Source: CAD feature listing. Evaluate the final solid. Frame: model axes, mm. Coordinates: 2 decimals unless noted, no trailing zeros. Order: outer loops, then holes, each group sorted by start corner. A loop starts at its lowest first (then second) coordinate and runs counter-clockwise, first axis right, second up.
```python
from build123d import *

# Parameters (mm, degrees)
SKETCH_R  = 1.8288
PAD_DEPTH = 3


with BuildPart() as part:
    # Sketch → Pad (new body)
    with BuildSketch(Plane.XY):
        with BuildLine():
            Line((0, 126), (0, 1))
            ThreePointArc((0, 1), (0.292893, 0.292893), (1, 0))
            Line((1, 0), (14.748, 0))
            ThreePointArc((14.748, 0), (15.455107, 0.292893), (15.748, 1))
            Line((15.748, 12.7), (15.748, 1))
            ThreePointArc((22.352, 12.7), (19.05, 16.002), (15.748, 12.7))
            Line((22.352, 12.7), (22.352, 1))
            ThreePointArc((22.352, 1), (22.644893, 0.292893), (23.352, 0))
            Line((23.352, 0), (150.6479, 0))
            ThreePointArc((150.6479, 0), (151.355007, 0.292893), (151.6479, 1))
            Line((151.6479, 12.7), (151.6479, 1))
            ThreePointArc((158.2519, 12.7), (154.9499, 16.002), (151.6479, 12.7))
            Line((158.2519, 12.7), (158.2519, 1))
            ThreePointArc((158.2519, 1), (158.544793, 0.292893), (159.2519, 0))
            Line((159.2519, 0), (286.5478, 0))
            ThreePointArc((286.5478, 0), (287.254907, 0.292893), (287.5478, 1))
            Line((287.5478, 12.7), (287.5478, 1))
            ThreePointArc((294.1518, 12.7), (290.8498, 16.002), (287.5478, 12.7))
            Line((294.1518, 12.7), (294.1518, 1))
            ThreePointArc((294.1518, 1), (294.444693, 0.292893), (295.1518, 0))
            Line((295.1518, 0), (308.8998, 0))
            ThreePointArc((308.8998, 0), (309.606907, 0.292893), (309.8998, 1))
            Line((309.8998, 1), (309.8998, 24.9))
            ThreePointArc((310.8998, 25.9), (310.192693, 25.607107), (309.8998, 24.9))
            Line((310.8998, 25.9), (330.9999, 25.9))
            ThreePointArc((330.9999, 25.9), (331.707007, 26.192893), (331.9999, 26.9))
            Line((331.9999, 26.9), (331.9999, 126))
            ThreePointArc((331.9999, 126), (331.707007, 126.707107), (330.9999, 127))
            Line((330.9999, 127), (1, 127))
            ThreePointArc((1, 127), (0.292893, 126.707107), (0, 126))
        make_face()
        with Locations((10.46, 120.65)):
            Circle(SKETCH_R, mode=Mode.SUBTRACT)
    extrude(amount=PAD_DEPTH)


solid = part.part
```
1. Pin query (flat end, axial travel): P1, Ø2, axis at x = 10.46, y = 120.65, coming from the +Z side. Return the tip coordinate at first contact, or that it passes through.
Findings:
P1: passes through
2. Section query B-B on x = 19.05. Return loops of the section in (y, z).
Findings:
outline: (16, 0) - (127, 0) - (127, 3) - (16, 3) - close
3. Ray query, line 1 (Y direction, x = 10.46, z = 1.7); line 2 (X direction, y = 120.65, z = 1.55); line 3 (X direction, y = 23, z = 0.9). Return the intervals inside material, ascending.
Findings:
line 1: y = 0 to 118.82, 122.48 to 127
line 2: x = 0 to 8.63, 12.29 to 332
line 3: x = 0 to 309.9
